CAD build for the part. Positions are in the model's coordinates, mm. A direction names the side the tool comes from. Coordinates: 2 decimals unless noted, no trailing zeros. Loops run counter-clockwise (first coordinate to the right, second up) from the corner with the lowest first, then second, coordinate; pieces in that order, holes last. Notation, with made-up numbers: (8.25, 39) -> (60.25, 39) arc R19 cw to (60.25, 55) -> close; hole circle Ø10 at (-14, -3.75). An arc over 180 degrees is marked (long way). Answer as a JSON object with one key per item and string values. Group by question number.
from build123d import *

# Parameters (mm, degrees)
BOSS_EXTRUDE1_DEPTH = 25
SKETCH3_R           = 4.8
CUT_EXTRUDE1_DEPTH  = 7.5
SKETCH6_W           = 2
SKETCH6_H           = 6.35
BOSS_EXTRUDE2_DEPTH = 90
FILLET2_R           = 1
SKETCH7_R           = 3.265
CUT_EXTRUDE2_DEPTH  = 55.212544674


with BuildPart() as part:
    # Sketch2 → Boss-Extrude1 (new body)
    with BuildSketch(Plane.XY):
        Polygon((18, 45), (18, 25), (18, -25), (18, -45), (33, -45), (33, 45), align=None)
    extrude(amount=BOSS_EXTRUDE1_DEPTH)

    # Sketch3 → Cut-Extrude1 (cut)
    with BuildSketch(Plane(origin=(18, 0, 0), x_dir=(0, 0, -1), z_dir=(1, 0, 0))):
        with Locations(Location((-12.5, 0, 0), (0, 0, 90))):
            Circle(SKETCH3_R)
    extrude(amount=CUT_EXTRUDE1_DEPTH, mode=Mode.SUBTRACT)

    # Sketch6 → Boss-Extrude2 (add, through all)
    with BuildSketch(Plane(origin=(0, 45, 0), x_dir=(1, 0, 0), z_dir=(0, 1, 0))):
        with Locations((34, -12.5)):
            Rectangle(SKETCH6_W, SKETCH6_H)
    extrude(amount=-BOSS_EXTRUDE2_DEPTH)

    # Fillet2
    fillet2_edges = [part.edges().sort_by_distance(p)[0] for p in [
        (33, 0, 9.325),
        (33, 0, 15.675),
    ]]
    fillet(fillet2_edges, radius=FILLET2_R)
    fillet2_2_edges = [part.edges().sort_by_distance(p)[0] for p in [
        (35, 0, 9.325),
        (35, 0, 15.675),
    ]]
    fillet(fillet2_2_edges, radius=FILLET2_R - 0.0001)  # a hair under: the kernel refuses the full size

    # Sketch7 → Cut-Extrude2 (cut, through all)
    with BuildSketch(Plane.ZY.offset(-18)):
        with Locations(Location((12.5, 35, 0), (0, 0, 270))):
            Circle(SKETCH7_R)
        with Locations(Location((12.5, -35, 0), (0, 0, 270))):
            Circle(SKETCH7_R)
    extrude(amount=-CUT_EXTRUDE2_DEPTH, mode=Mode.SUBTRACT)


solid = part.part
Item 1: Band-saw the part on A-A, the plane z = 12.5. List the corners of the cut face in (x, y) (3 decimals), and give its area (3 significant figures).
Item 2: Pull direction Z, two halves, no side cores. Call faces 4 (the flat face through (25.5, 0, 13)), 5 (the flat face through (26, -45, 12)), 6 (the flat face through (25, 1, 0)): +Z half, -Z half, draft (parallel to the pull), parting line (faces both ways), or undercut.
Item 3: Band-saw the part on B-B, the plane y = -35. List the corners of the cut face in (x, z) (3 decimals).
Item 4: Band-saw the part on C-C, the plane x = 29.5. List the corners of the cut face in (y, z) (3 decimals), and give its area (3 significant figures).
Item 5: Flat gauge pins, fed straight in: P1, Ø6.5, axis at y = 8.5, z = 4.5, coming from the +X side; P2, Ø6, axis at y = 35, z = 12.5, coming from the -X side. Where does each tip first touch, or does it go through?
Item 6: Drill centre lines: L1, parallel to Y at x = 26.25, z = 12.5 (3 decimals); L2, parallel to Z at x = 29.5, y = -35 (3 decimals); L3, parallel to X at y = 17, z = 23.75. Where is each one in solid material? Low to high.
Item 7: 3-axis set-ups, long thin cutter, end or side, ignore diameter. For faces 1 (the flat face through (33, -1, 4)), 2 (the flat face through (33, -1, 21)), 3 (the cylindrical face through (21.7, 2.58, 16.55)): which of +Z, -Z, +X, -X, +Y, -Y reach the whole face in a straight line?
Reply:
{
 "1": {"outline": "(18, -45) -> (35, -45) -> (35, -38.265) -> (18, -38.265) -> close; (18, -31.735) -> (35, -31.735) -> (35, 31.735) -> (18, 31.735) -> (18, 4.8) -> (25.5, 4.8) -> (25.5, -4.8) -> (18, -4.8) -> close; (18, 38.265) -> (35, 38.265) -> (35, 45) -> (18, 45) -> close", "area": "1,240 mm²"},
 "2": {"face 4": "undercut", "face 5": "draft", "face 6": "-Z half"},
 "3": {"outline": "(18, 0) -> (33, 0) -> (33, 8.325) arc R1 cw to (33.585, 9.235) -> (18, 9.235) -> close; (18, 15.765) -> (33.585, 15.765) arc R1 cw to (33, 16.675) -> (33, 25) -> (18, 25) -> close"},
 "4": {"outline": "(-45, 0) -> (45, 0) -> (45, 25) -> (-45, 25) -> close; hole circle Ø6.53 at (-35, 12.5); hole circle Ø6.53 at (35, 12.5)", "area": "2,180 mm²"},
 "5": {"P1": "x = 33", "P2": "through"},
 "6": {"L1": "-45 to -38.265, -31.735 to 31.735, 38.265 to 45", "L2": "0 to 9.235, 15.765 to 25", "L3": "18 to 33"},
 "7": {"face 1": "-Z, +X, +Y, -Y", "face 2": "+Z, +X, +Y, -Y", "face 3": "-X"}
}
